Check sheet for the modelled part. Datum: model origin and axes. Units: mm. A direction names the side the tool comes from. Give positions to 0.01 mm unless a question says otherwise; leave off trailing zeros. Order: outer loops, then holes, each group sorted by start corner. A loop starts at its lowest first (then second) coordinate and runs counter-clockwise, first axis right, second up.
Autodesk Inventor part; units mm, degrees
ref_plane "YZ Plane" through (0, 0, 0) normal (1, 0, 0) x (0, 1, 0)
ref_plane "XZ Plane" through (0, 0, 0) normal (0, 1, 0) x (-1, 0, 0)
ref_plane "XY Plane" through (0, 0, 0) normal (0, 0, 1) x (1, 0, 0)
sketch "Sketch1" plane through (0, 0, 0) normal (0, 1, 0) x (-1, 0, 0)
  circle A0 centre (0, 0) radius 1.5875
  dimension "d0" = 3.175
extrude "Extrusion1" add sketch "Sketch1" along normal blind 6.858
sketch "Sketch2" plane through (0, 0, 0) normal (0, -1, 0) x (1, 0, 0)
  circle A0 centre (0, 0) radius 2.54
  dimension "d3" = 5.08
extrude "Extrusion2" add sketch "Sketch2" along normal blind 3.175
sketch "Sketch3" plane through (0, -3.175, 0) normal (0, -1, 0) x (1, 0, 0)
  line L0 (1.8331, 0) -> (0.9165, -1.5875)
  line L1 (0.9165, -1.5875) -> (-0.9165, -1.5875)
  line L2 (-0.9165, -1.5875) -> (-1.8331, 0)
  line L3 (-1.8331, 0) -> (-0.9165, 1.5875)
  line L4 (-0.9165, 1.5875) -> (0.9165, 1.5875)
  line L5 (0.9165, 1.5875) -> (1.8331, 0)
  point P0 (0, 0)
  point P1 (0, 0)
  dimension "d6" = 3.175
extrude "Extrusion3" cut sketch "Sketch3" against normal blind 1.905
thread "Thread1"
properties part number "Slide rod set screw" material "Steel, Galvanized"
(1) Cross-section at D-D on z = 2.1. Enter the section's corners in (x, y) (3 decimals), then the cut area to 3 significant figures.
Response values:
outline: (-1.429, -3.175) - (1.429, -3.175) - (1.429, 0) - (-1.429, 0) - close
area: 9.07 mm2
(2) Cross-section at B-B on y = 2.25. Enter the section's corners in (x, z) (1 decimal).
Response values:
outline: circle Ø3.2 at (0, 0)
(3) Release check for a two-part mould opening along X. For faces 4 (the face through (0, 6.858, 0)), 5 (the face through (0, -1.27, 0)), 6 (the face through (-0.33, -1.57, -2.52)) record: released by +X, released by -X, zero draft, split by the parting line, or undercut.
Response values:
face 4: zero draft
face 5: undercut
face 6: split by the parting line
(4) Gauge pin test, flat ends, axial feed: pin 1 Ø2 at (x, y) = (-0.5, -2) entering from -Z; pin 2 Ø1 at (y, z) = (3, -1.5) entering from -X; pin 3 Ø1.5 at (y, z) = (-1, 1) entering from +X. Record the tip position at first contact, or that the pin passes through.
Response values:
pin 1: stops at z = -2.54
pin 2: stops at x = -1.23
pin 3: stops at x = 2.53
(5) Material ranges on L1, parallel to Z at x = 0, y = 6; L2, parallel to Y at x = -1.9, z = 1.35 (3 decimals); L3, parallel to Y at x = -1.2, z = -0.95, recorded low to high.
Response values:
L1: z = -1.59 to 1.59
L2: y = -3.175 to 0
L3: y = -1.27 to 6.86
(6) Cross-section at A-A on x = 0. Enter the section's corners in (y, z) (1 decimal), then the cut area to 3 significant figures.
Response values:
outline: (-3.2, -2.5) - (0, -2.5) - (0, -1.6) - (6.9, -1.6) - (6.9, 1.6) - (0, 1.6) - (0, 2.5) - (-3.2, 2.5) - (-3.2, 1.6) - (-1.3, 1.6) - (-1.3, -1.6) - (-3.2, -1.6) - close
area: 31.9 mm2
(7) Set-up check for faces 1 (the face through (0.34, 3.38, 1.55)), 2 (the face through (0, -3.175, -2)), 3 (the face through (0, -2, -1.588)): record each of +Z, -Z, +X, -X, +Y, -Y from which the full face is reachable in a straight line by a thin tool's end or side.
Response values:
face 1: +Y
face 2: +Z, -Z, +X, -X, -Y
face 3: -Y
(8) Cross-section at C-C on z = 0.7. Enter the section's corners in (x, y) (3 decimals).
Response values:
outline: (-2.442, -3.175) - (-1.429, -3.175) - (-1.429, -1.27) - (1.429, -1.27) - (1.429, -3.175) - (2.442, -3.175) - (2.442, 0) - (1.425, 0) - (1.425, 6.858) - (-1.425, 6.858) - (-1.425, 0) - (-2.442, 0) - close
